For this review, take the finished solid that the model builds, in its own axes (mm). Give positions to 0.01 mm unless a question says otherwise; leave off trailing zeros. Loops run counter-clockwise (first coordinate to the right, second up) from the corner with the lowest first, then second, coordinate; pieces in that order, holes last. Notation, with made-up numbers: (0, -39.5) - (35, -39.5) arc R26 cw to (35, -13.5) - close; hole circle Ø3 at (78, 61.5). An arc over 180 degrees is marked (long way). Answer in a Markdown table with one row per item.
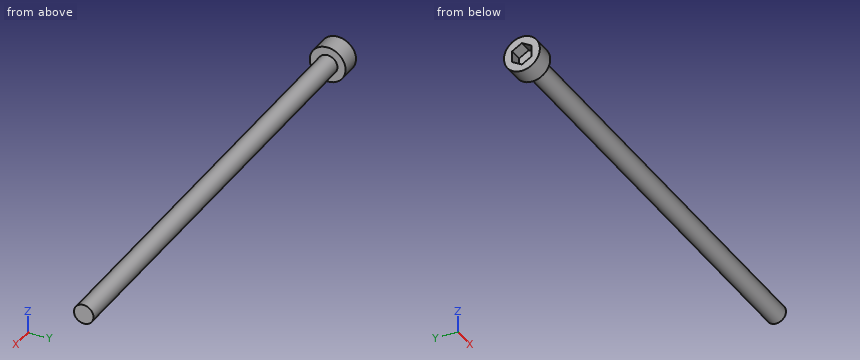
```python
from build123d import *

# Parameters (mm, degrees)
F0_R     = 2.75
F1_DEPTH = 2
F2_R     = 2.75
F3_DEPTH = 1
F4_R     = 1.5
F5_DEPTH = 70


with BuildPart() as f1:
    # F0 (on Right) → F1 (new body)
    with BuildSketch(Plane.YZ):
        Circle(F0_R)
        Polygon((-1.5, -0.866025), (-1.5, 0.866025), (0, 1.732051), (1.5, 0.866025), (1.5, -0.866025), (0, -1.732051), align=None, mode=Mode.SUBTRACT)
    extrude(amount=F1_DEPTH)

    # F2 (on face) → F3 (join)
    with BuildSketch(Plane.YZ.offset(2)):
        Circle(F2_R)
    extrude(amount=F3_DEPTH)

    # F4 (on face) → F5 (join)
    with BuildSketch(Plane.YZ.offset(3)):
        Circle(F4_R)
    extrude(amount=F5_DEPTH)


solid = f1.part
```
1. We need section A-A, the plane z = 0. Give the boundary of the cut face in (x, y).
Values:
| item | result |
|---|---|
| outline | (0, -2.75) - (3, -2.75) - (3, -1.5) - (73, -1.5) - (73, 1.5) - (3, 1.5) - (3, 2.75) - (0, 2.75) - (0, 1.5) - (2, 1.5) - (2, -1.5) - (0, -1.5) - close |
2. Wall thickness on line 1 (Z direction, x = 38, y = -0.15); line 2 (X direction, y = -1.7, z = 0.35); line 3 (X direction, y = 0, z = 0): over which ranges is each line inside the solid? List them lowest first. Write a range as [from, to].
Values:
| item | result |
|---|---|
| line 1 | z = [-1.49, 1.49] |
| line 2 | x = [0, 3] |
| line 3 | x = [2, 73] |
3. We need section B-B, the plane x = 13. Give the boundary of the cut face in (y, z), and give its area (3 significant figures).
Values:
| item | result |
|---|---|
| outline | circle Ø3 at (0, 0) |
| area | 7.07 mm^2 |
4. Clearance check with a flat-ended pin moving along its axis: pin 1 (1 mm diameter, centred on x = 58.5, y = 0.5, fed in from -Z). State where the tip first meets the part, or that it passes through.
Values:
| item | result |
|---|---|
| pin 1 | stops at z = -1.5 |
